Check sheet for the drawn part. Datum: minimum x, y, z corner. Units: mm. A direction names the side the tool comes from. Give positions to 0.01 mm unless a question says otherwise; leave off trailing zeros. Loops run counter-clockwise (first coordinate to the right, second up) from the corner with the lowest first, then second, coordinate; pieces in that order, holes last.
1. Cross-section at A-A, the plane x = 17. Record the cut outline in (y, z).
2. Tool access check on the marked faces 4, 5 and 6. Record the directions out of +Z, -Z, +X, -X, +Y, -Y that give a thin tool (end or side, any length) a straight path to the whole face; none if there is none.
3. Release check for a two-part mould opening along Z. For the marked faces 1, 2 and 3 record: +Z half, -Z half, draft (parallel to the pull), parting line (faces both ways), or undercut.
4. Cross-section at B-B, the plane z = 5.5. Record the cut outline in (x, y).
5. Cross-section at D-D, the plane z = 8.5. Record the cut outline in (x, y).
6. Cross-section at C-C, the plane y = 17.75. Record the cut outline in (x, z).
7. Go/stop test with flat-tipped pins: pin 1 Ø5 at (y, z) = (18, 4.5) entering from -X; pin 2 Ø4.5 at (x, z) = (5, 5) entering from +Y; pin 3 Ø5 at (y, z) = (19.5, 6.5) entering from +X. Record where each tip stops, or that it passes through.
8. Material ranges on L1, parallel to Y at x = 17, z = 3.5; L2, parallel to X at y = 2.4, z = 5; L3, parallel to X at y = 15.25, z = 7.25, recorded low to high.
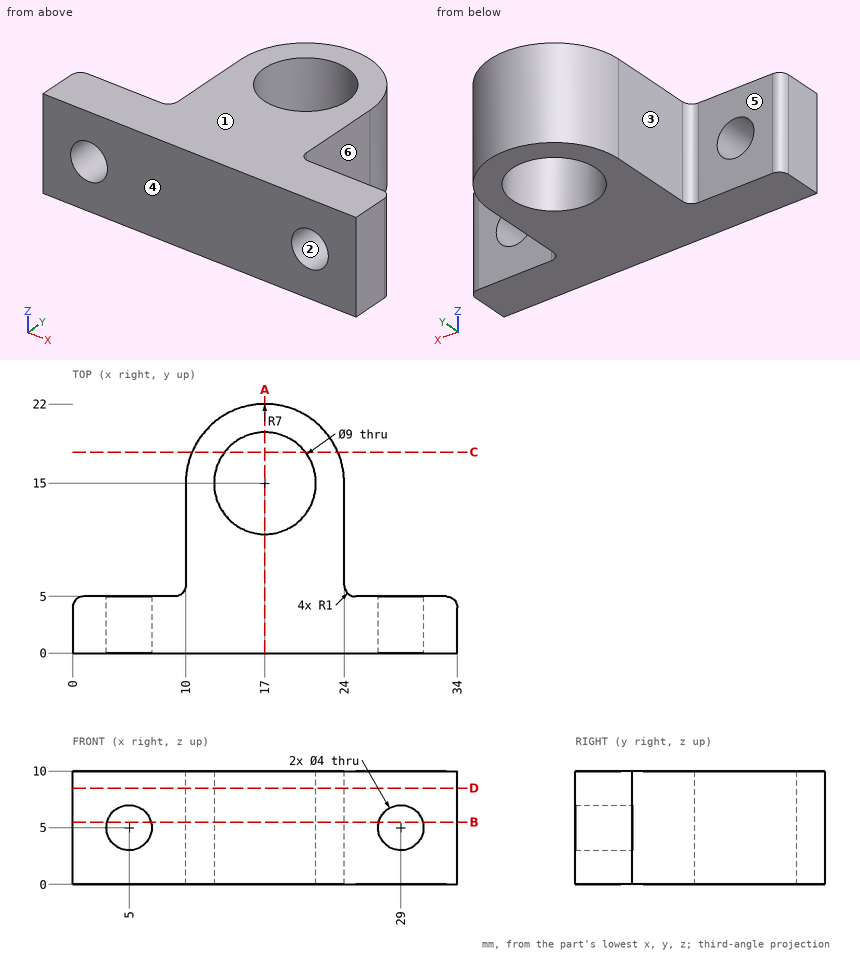
Result:
1. outline: (0, 0) - (10.5, 0) - (10.5, 10) - (0, 10) - close; (19.5, 0) - (22, 0) - (22, 10) - (19.5, 10) - close
2. face 4: +Z, -Z, +X, -X, -Y
2. face 5: +Z, -Z, -X, +Y
2. face 6: +Z, -Z, +X, +Y
3. face 1: +Z half
3. face 2: undercut
3. face 3: draft
4. outline: (0, 0) - (3.06, 0) - (3.06, 5) - (1, 5) arc R1 ccw to (0, 4) - close; (6.94, 0) - (27.06, 0) - (27.06, 5) - (25, 5) arc R1 cw to (24, 6) - (24, 15) arc R7 ccw to (10, 15) - (10, 6) arc R1 cw to (9, 5) - (6.94, 5) - close; (30.94, 0) - (34, 0) - (34, 4) arc R1 ccw to (33, 5) - (30.94, 5) - close; hole circle Ø9 at (17, 15)
5. outline: (0, 0) - (34, 0) - (34, 4) arc R1 ccw to (33, 5) - (25, 5) arc R1 cw to (24, 6) - (24, 15) arc R7 ccw to (10, 15) - (10, 6) arc R1 cw to (9, 5) - (1, 5) arc R1 ccw to (0, 4) - close; hole circle Ø9 at (17, 15)
6. outline: (10.56, 0) - (13.44, 0) - (13.44, 10) - (10.56, 10) - close; (20.56, 0) - (23.44, 0) - (23.44, 10) - (20.56, 10) - close
7. pin 1: stops at x = 10.02
7. pin 2: stops at y = 5
7. pin 3: stops at x = 23.71
8. L1: y = 0 to 10.5, 19.5 to 22
8. L2: x = 0 to 3, 7 to 27, 31 to 34
8. L3: x = 10 to 12.51, 21.49 to 24
